```python
from build123d import *

# Parameters (mm, degrees)
F0_W     = 139.7
F0_H     = 88.9
F0_W_2   = 127
F0_H_2   = 76.2
F1_DEPTH = 76.2
F2_W     = 63.5
F2_H     = 25.4
F3_DEPTH = 166.37
F4_R     = 12.7
F5_DEPTH = 213.36


with BuildPart() as f1:
    # F0 (on Top) → F1 (new body)
    with BuildSketch(Plane.XY):
        Rectangle(F0_W, F0_H)
        Rectangle(F0_W_2, F0_H_2, mode=Mode.SUBTRACT)
    extrude(amount=F1_DEPTH)

    # F2 (on face) → F3 (cut)
    with BuildSketch(Plane.XZ.offset(44.45)):
        with Locations((0, 63.5)):
            Rectangle(F2_W, F2_H)
    extrude(amount=-F3_DEPTH, mode=Mode.SUBTRACT)

    # F4 (on face) → F5 (cut)
    with BuildSketch(Plane.YZ.offset(69.85)):
        with Locations((0, 38.1)):
            Circle(F4_R)
    extrude(amount=-F5_DEPTH, mode=Mode.SUBTRACT)


solid = f1.part
```
Input: part model. Units: mm. Frame: model coordinates. A direction names the side the tool comes from. Give positions to 0.01 mm unless a question says otherwise; leave off trailing zeros. Order: outer loops, then holes, each group sorted by start corner. A loop starts at its lowest first (then second) coordinate and runs counter-clockwise, first axis right, second up.
1. Cut plane A-A (z = 38.1). Return loops of the section in (x, y).
Computed:
outline: (-69.85, -44.45) - (69.85, -44.45) - (69.85, -12.7) - (63.5, -12.7) - (63.5, -38.1) - (-63.5, -38.1) - (-63.5, -12.7) - (-69.85, -12.7) - close; (-69.85, 12.7) - (-63.5, 12.7) - (-63.5, 38.1) - (63.5, 38.1) - (63.5, 12.7) - (69.85, 12.7) - (69.85, 44.45) - (-69.85, 44.45) - close
2. Cut plane D-D (y = 0). Return loops of the section in (x, z).
Computed:
outline: (-69.85, 0) - (-63.5, 0) - (-63.5, 25.4) - (-69.85, 25.4) - close; (-69.85, 50.8) - (-63.5, 50.8) - (-63.5, 76.2) - (-69.85, 76.2) - close; (63.5, 0) - (69.85, 0) - (69.85, 25.4) - (63.5, 25.4) - close; (63.5, 50.8) - (69.85, 50.8) - (69.85, 76.2) - (63.5, 76.2) - close
3. Cut plane C-C (x = -38). Return loops of the section in (y, z), and give its area (3 significant figures).
Computed:
outline: (-44.45, 0) - (-38.1, 0) - (-38.1, 76.2) - (-44.45, 76.2) - close; (38.1, 0) - (44.45, 0) - (44.45, 76.2) - (38.1, 76.2) - close
area: 968 mm2
4. Set-up query: faces 4 (the face through (31.75, -41, 63)), 5 (the face through (63.5, -17, 38)), 6 (the face through (69.85, -11, 29)). Return all of +Z, -Z, +X, -X, +Y, -Y with unobstructed straight access to the full face (end or side cutting, diameter ignored); none if empty.
Computed:
face 4: +Z, +Y, -Y
face 5: +Z, -Z
face 6: +Z, -Z, +X, +Y, -Y
5. Cut plane B-B (y = 35). Return loops of the section in (x, z).
Computed:
outline: (-69.85, 0) - (-63.5, 0) - (-63.5, 76.2) - (-69.85, 76.2) - close; (63.5, 0) - (69.85, 0) - (69.85, 76.2) - (63.5, 76.2) - close
6. Pin query (flat end, axial travel): pin 1 Ø1.9 at (x, y) = (-5.5, 43) entering from +Z. Return the tip coordinate at first contact, or that it passes through.
Computed:
pin 1: stops at z = 50.8
7. Draft query along X for faces 1 (the face through (-64, 1, 76.2)), 2 (the face through (31.75, 41, 63)), 3 (the face through (-69.85, -11, 29)). Return one class per face: released by +X, released by -X, zero draft, split by the parting line, or undercut.
Computed:
face 1: zero draft
face 2: undercut
face 3: released by -X
8. Line query: probe 1 along X at (y, z) = (17, 23); probe 2 along Y at (x, z) = (68, 38); probe 3 along Y at (x, z) = (-42, 39.5). Output: solid intervals per line, ascending.
Computed:
probe 1: x = -69.85 to -63.5, 63.5 to 69.85
probe 2: y = -44.45 to -12.7, 12.7 to 44.45
probe 3: y = -44.45 to -38.1, 38.1 to 44.45
